from build123d import *

# Parameters (mm, degrees)
SKETCH_R           = 6
PAD_DEPTH          = 4
SKETCH001_R        = 12.5
PAD001_DEPTH       = 3
SKETCH002_R        = 4
POCKET_DEPTH       = 3
POLARPATTERN_COUNT = 5
FILLET_R           = 2
SKETCH003_R        = 2.31
POCKET001_DEPTH    = 3
POCKET001_FACE25_R = 6
POCKET002_DEPTH    = 1
POCKET002_FACE26_R = 2.31
POCKET003_DEPTH    = 1.5
POCKET003_FACE26_R = 2.31
POCKET004_DEPTH    = 1.501
SKETCH005_R        = 6
SKETCH005_R_2      = 2.31
PAD002_DEPTH       = 3


with BuildPart() as part:
    # Sketch → Pad (new body)
    with BuildSketch(Plane.XY):
        Circle(SKETCH_R)
        Polygon((-2.286307, -3.96), (2.286307, -3.96), (4.572614, 0), (2.286307, 3.96), (-2.286307, 3.96), (-4.572614, 0), align=None, mode=Mode.SUBTRACT)
    extrude(amount=PAD_DEPTH)

    # Sketch001 (on Face9 of Pad) → Pad001 (join)
    with BuildSketch(Plane.XY.offset(4)):
        Circle(SKETCH001_R)
    extrude(amount=PAD001_DEPTH)

    # Sketch002 (on Face3 of Pad001) → Pocket (cut)
    with BuildSketch(Plane.XY.offset(7)):
        with Locations((0, 12.5)):
            Circle(SKETCH002_R)
    pocket = extrude(amount=-POCKET_DEPTH, mode=Mode.SUBTRACT)

    # PolarPattern: Pocket ×5 about axis
    polarpattern_axis = Axis((0, 0, 0), (0, 0, 1))
    for i in range(1, POLARPATTERN_COUNT):
        add(pocket.rotate(polarpattern_axis, i * 360 / POLARPATTERN_COUNT), mode=Mode.SUBTRACT)

    # Fillet
    fillet_edges = [part.edges().sort_by_distance(p)[0] for p in [
        (-12.499674, -0.090275, 5.5),
        (-10.059387, 7.420158, 5.5),
        (-3.948468, 11.86, 5.5),
        (3.948468, 11.86, 5.5),
        (-3.776755, -11.915793, 5.5),
        (-10.165511, -7.27409, 5.5),
        (10.165511, -7.27409, 5.5),
        (3.776755, -11.915793, 5.5),
        (10.059387, 7.420158, 5.5),
        (12.499674, -0.090275, 5.5),
    ]]
    fillet(fillet_edges, radius=FILLET_R)

    # Sketch003 (on Face31 of Fillet) → Pocket001 (cut)
    with BuildSketch(Plane(origin=(0, 0, 4), x_dir=(1, 0, 0), z_dir=(0, 0, -1))):
        Circle(SKETCH003_R)
    extrude(amount=-POCKET001_DEPTH, mode=Mode.SUBTRACT)

    # Pocket001 Face25 → Pocket002 (cut)
    with BuildSketch(Plane(origin=(0, 0, 0), x_dir=(0, -1, 0), z_dir=(0, 0, -1))):
        Circle(POCKET001_FACE25_R)
        Polygon((0, 4.572614), (3.96, 2.286307), (3.96, -2.286307), (0, -4.572614), (-3.96, -2.286307), (-3.96, 2.286307), align=None, mode=Mode.SUBTRACT)
    extrude(amount=-POCKET002_DEPTH, mode=Mode.SUBTRACT)

    # Pocket002 Face26 → Pocket003 (cut)
    with BuildSketch(Plane(origin=(0, 0, 4), x_dir=(0, -1, 0), z_dir=(0, 0, -1))):
        Polygon((0, 4.572614), (-3.96, 2.286307), (-3.96, -2.286307), (0, -4.572614), (3.96, -2.286307), (3.96, 2.286307), align=None)
        Circle(POCKET002_FACE26_R, mode=Mode.SUBTRACT)
    extrude(amount=-POCKET003_DEPTH, mode=Mode.SUBTRACT)

    # Pocket003 Face26 → Pocket004 (cut, through all)
    with BuildSketch(Plane(origin=(0, 0, 5.5), x_dir=(0, -1, 0), z_dir=(0, 0, -1))):
        Polygon((0, 4.572614), (-3.96, 2.286307), (-3.96, -2.286307), (0, -4.572614), (3.96, -2.286307), (3.96, 2.286307), align=None)
        Circle(POCKET003_FACE26_R, mode=Mode.SUBTRACT)
    extrude(amount=-POCKET004_DEPTH, mode=Mode.SUBTRACT)

    # Sketch005 (on Face30 of Pocket004) → Pad002 (join)
    with BuildSketch(Plane(origin=(0, 0, 1), x_dir=(1, 0, 0), z_dir=(0, 0, -1))):
        Circle(SKETCH005_R)
        Circle(SKETCH005_R_2, mode=Mode.SUBTRACT)
    extrude(amount=-PAD002_DEPTH)


solid = part.part
Geometry: final body of the model. Coordinates: model frame, mm. A direction names the side the tool comes from. Give positions to 0.01 mm unless a question says otherwise; leave off trailing zeros. Loops run counter-clockwise (first coordinate to the right, second up) from the corner with the lowest first, then second, coordinate; pieces in that order, holes last. Notation, with made-up numbers: M -4,30.25 L 2,30.25 A21 ccw 2,45.25 Z; hole C 56.5,41 d3. An arc over 180 degrees is marked long. Put each result on its own line as item: value. Start each with the question number.
1) Cut plane D-D (x = -6.75). Output: boundary loops of the cut face in (y, z).
2) Cut plane A-A (x = 0). Output: boundary loops of the cut face in (y, z), then the cut area to 3 significant figures.
3) Cut plane C-C (y = 3.25). Output: boundary loops of the cut face in (x, z).
4) Pull-direction query (X, two-part tool) for faces 1 (the cylindrical face through (11.881, -3.884, 5.479)), 2 (the cylindrical face through (2.2, -0.7, 2.5)), 3 (the flat face through (0, 3.96, 5)), 4 (the flat face through (3, -6, 4)); classes: pulls with the +X half, pulls with the -X half, needs draft (parallel to the pull), parting line crosses it, or undercut.
5) Ray query, line 1 along Y through (x, z) = (0, 2.65); line 2 along Y through (x, z) = (1, 1.75); line 3 along Z through (x, y) = (1.5, 2.25). Return the intervals inside material, ascending.
6) Cut plane B-B (z = 2). Output: boundary loops of the cut face in (x, y).
7) Contact query for flat-ended pins moving along their axis: pin 1 (10 mm diameter, centred on x = 8.5, y = 2, fed in from +Z); pin 2 (0.9 mm diameter, centred on x = 1, z = 5, fed in from -Y); pin 3 (4 mm diameter, centred on x = 0, y = 0, fed in from +Z); pin 4 (3.5 mm diameter, centred on x = -0.5, z = 5.5, fed in from +Y). Output: stop coordinate, or through.
8) Access query for faces 5 (the cylindrical face through (8.067, 2.68, 5.521)), 6 (the cylindrical face through (5.723, 1.802, 2.479)), 7 (the flat face through (2, -2, 4)). Directions: +Z, -Z, +X, -X, +Y, -Y. A direction counts if a zero-diameter tool reaches every point of the face in a straight line with its end or side. Return the directions, or none.
Verdict:
1. outline: M -6.16,4 L 10.52,4 L 10.52,7 L -6.16,7 Z
2. outline: M -12.5,4 L -6,4 L -6,1 L -2.31,1 L -2.31,4 L -3.96,4 L -3.96,7 L -12.5,7 Z; M 2.31,1 L 6,1 L 6,4 L 8.5,4 L 8.5,7 L 3.96,7 L 3.96,4 L 2.31,4 Z
2. area: 61.4 mm2
3. outline: M -7.94,4 L -5.04,4 L -5.04,1 L 5.04,1 L 5.04,4 L 7.94,4 L 7.94,7 L 2.7,7 L 2.7,4 L -2.7,4 L -2.7,7 L -7.94,7 Z
4. face 1: pulls with the +X half
4. face 2: undercut
4. face 3: undercut
4. face 4: needs draft
5. line 1: -6 to -2.31, 2.31 to 6
5. line 2: -5.92 to -2.08, 2.08 to 5.92
5. line 3: 1 to 4
6. outline: C 0,0 d12; hole C 0,0 d4.62
7. pin 1: z = 7
7. pin 2: y = -12.49
7. pin 3: through
7. pin 4: y = 9.19
8. face 5: +Z, -Z, +X
8. face 6: -Z
8. face 7: +Z
